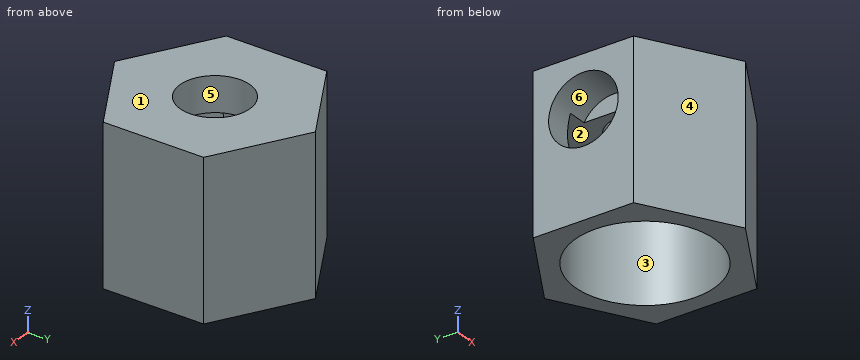
```python
from build123d import *

# Parameters (mm, degrees)
BOSS_EXTRUDE1_DEPTH = 6
SKETCH3_R           = 2
CUT_EXTRUDE1_DEPTH  = 2.5
CUT_EXTRUDE5_REACH  = 11.713
SKETCH5_R           = 2
SKETCH6_R           = 2
BOSS_EXTRUDE2_DEPTH = 3
SKETCH7_R           = 4
CUT_EXTRUDE6_DEPTH  = 7


with BuildPart() as part:
    # Sketch2 → Boss-Extrude1 (new body)
    with BuildSketch(Plane.XY):
        Polygon((0, -5.773502692), (5, -2.886751346), (5, 2.886751346), (0, 5.773502692), (-5, 2.886751346), (-5, -2.886751346), align=None)
    extrude(amount=BOSS_EXTRUDE1_DEPTH)

    # Sketch3 → Cut-Extrude1 (cut)
    with BuildSketch(Plane.ZY.offset(5)):
        with Locations(Location((3, 0, 0), (0, 0, 270))):
            Circle(SKETCH3_R)
    extrude(amount=-CUT_EXTRUDE1_DEPTH, mode=Mode.SUBTRACT)

    # Sketch5 → Cut-Extrude5 (cut, up to next)
    with BuildSketch(Plane.XY.offset(6), mode=Mode.PRIVATE) as cut_extrude5_sk1:
        Circle(SKETCH5_R)
    cut_extrude5_tool1 = extrude(cut_extrude5_sk1.sketch, amount=-CUT_EXTRUDE5_REACH, mode=Mode.PRIVATE) & part.part
    add(cut_extrude5_tool1.solids().sort_by_distance((0, 0, 6))[0], mode=Mode.SUBTRACT)

    # Sketch6 → Boss-Extrude2 (add)
    with BuildSketch(Plane(origin=(0, 0, 0), x_dir=(-1, 0, 0), z_dir=(0, 0, -1))):
        Polygon((0, 5.773502692), (-5, 2.886751346), (-5, -2.886751346), (0, -5.773502692), (5, -2.886751346), (5, 2.886751346), align=None)
        with Locations(Location((0, 0, 0), (0, 0, 180))):
            Circle(SKETCH6_R, mode=Mode.SUBTRACT)
    extrude(amount=BOSS_EXTRUDE2_DEPTH)

    # Sketch7 → Cut-Extrude6 (cut)
    with BuildSketch(Plane(origin=(0, 0, -3), x_dir=(-1, 0, 0), z_dir=(0, 0, -1))):
        Circle(SKETCH7_R)
    extrude(amount=-CUT_EXTRUDE6_DEPTH, mode=Mode.SUBTRACT)


solid = part.part
```
Geometry check sheet. Reference: the model listing, model coordinates, mm. Face numbers are marked on the shaded views. A direction names the side the tool comes from. Give positions to 0.01 mm unless a question says otherwise; leave off trailing zeros. Order: outer loops, then holes, each group sorted by start corner. A loop starts at its lowest first (then second) coordinate and runs counter-clockwise, first axis right, second up.
1. Section check A-A, the plane y = 0. Enter the section's corners in (x, z), and give its area (3 significant figures).
2. Section check D-D, the plane z = 5.25. Enter the section's corners in (x, y).
3. Section check B-B, the plane z = 0.25. Enter the section's corners in (x, y), and give its area (3 significant figures).
4. Section check C-C, the plane x = 1.5. Enter the section's corners in (y, z).
5. Release check for a two-part mould opening along X. For the marked faces 1, 2, 3 and 4 record: pulls with the +X half, pulls with the -X half, needs draft (parallel to the pull), parting line crosses it, or undercut.
6. Access from +Z, -Z, +X, -X, +Y, -Y to the whole of each face (thin tool, end or side, straight path). Record for the marked faces 5 and 6.
7. Thickness scan on L1, parallel to X at y = 1, z = 5.5; L2, parallel to Z at x = 2.75, y = -2.5; L3, parallel to Z at x = -4.45, y = 0. Record the ranges inside material, lowest first.
8. Gauge pin test, flat end, axial feed: pin 1 Ø1.5 at (x, z) = (-0.5, 3.5) entering from +Y. Record the tip position at first contact, or that the pin passes through.
Values follow:
1. outline: (-5, -3) - (-4, -3) - (-4, 1) - (-5, 1) - close; (-5, 5) - (-2.5, 5) - (-2.5, 4) - (-2, 4) - (-2, 6) - (-5, 6) - close; (2, 4) - (4, 4) - (4, -3) - (5, -3) - (5, 6) - (2, 6) - close
1. area: 20.5 mm2
2. outline: (-5, -2.89) - (0, -5.77) - (5, -2.89) - (5, 2.89) - (0, 5.77) - (-5, 2.89) - close; hole circle Ø4 at (0, 0)
3. outline: (-5, -2.89) - (0, -5.77) - (5, -2.89) - (5, 2.89) - (0, 5.77) - (-5, 2.89) - close; hole circle Ø8 at (0, 0)
3. area: 36.3 mm2
4. outline: (-4.91, -3) - (-3.71, -3) - (-3.71, 4) - (-1.32, 4) - (-1.32, 6) - (-4.91, 6) - close; (1.32, 4) - (3.71, 4) - (3.71, -3) - (4.91, -3) - (4.91, 6) - (1.32, 6) - close
5. face 1: needs draft
5. face 2: undercut
5. face 3: undercut
5. face 4: pulls with the -X half
6. face 5: +Z, -Z
6. face 6: -X
7. L1: x = -5 to -1.73, 1.73 to 5
7. L2: z = 4 to 6
7. L3: z = -3 to 1, 5 to 6
8. pin 1: stops at y = 5.77
